Geometry check sheet. Reference: drawing and pictorial views, mm from the part's lowest x, y, z. Give positions to 0.01 mm unless a question says otherwise; leave off trailing zeros. Write each loop counter-clockwise with the first axis right and the second up, starting at its lowest first coordinate (ties: lowest second). Pieces come first, ordered by that corner, then holes. Notation, with made-up numbers: M 24.5,-33.75 L 65.5,-33.75 A19 ccw 65.5,2.25 Z; hole C 37.25,64.5 d10. An arc over 180 degrees is marked long. Answer as a JSON object with one key per item and string values.
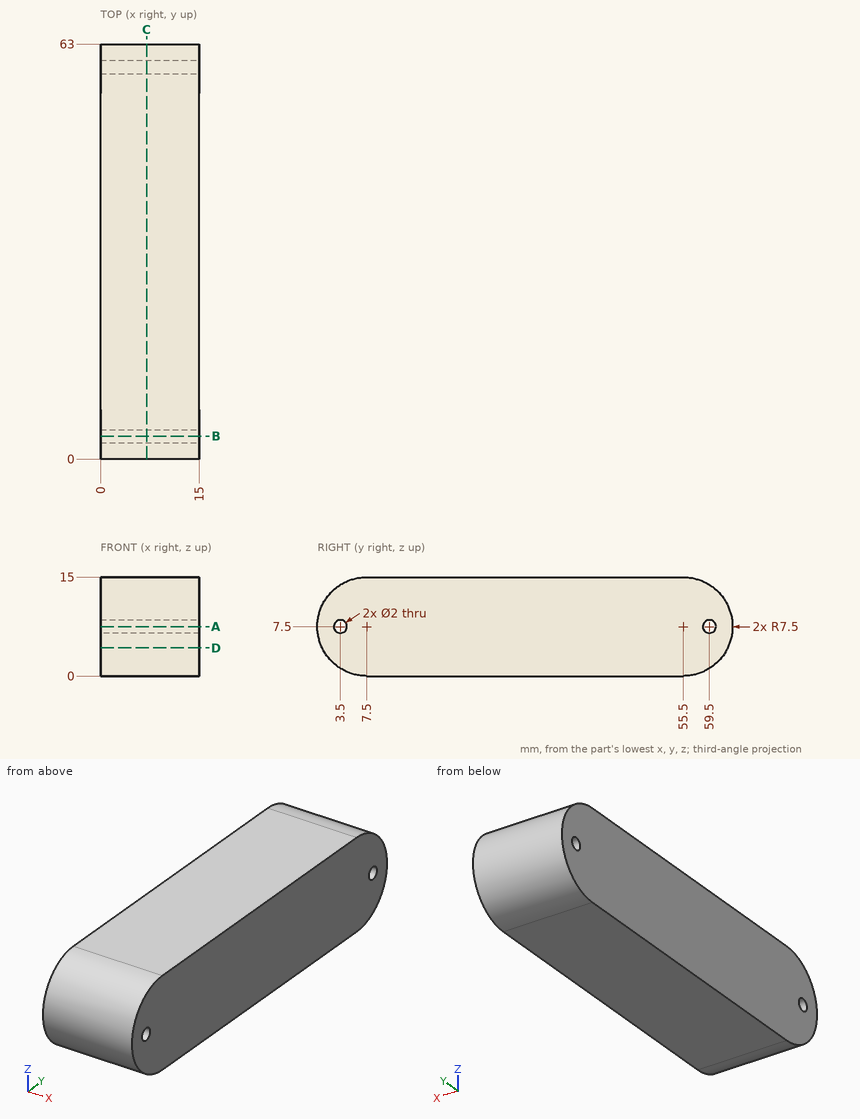
1) Section check C-C on x = 7. Record the boundary of the cut face in (y, z), and give its area (3 significant figures).
Completed:
{"outline": "M 7.5,0 L 55.5,0 A7.5 ccw 55.5,15 L 7.5,15 A7.5 ccw Z; hole C 3.5,7.5 d2; hole C 59.5,7.5 d2", "area": "890 mm2"}
2) Section check A-A on z = 7.5. Record the boundary of the cut face in (x, y).
Completed:
{"outline": "M 0,0 L 15,0 L 15,2.5 L 0,2.5 Z; M 0,4.5 L 15,4.5 L 15,58.5 L 0,58.5 Z; M 0,60.5 L 15,60.5 L 15,63 L 0,63 Z"}
3) Go/stop test with a flat-tipped pin: pin 1 (3 mm diameter, centred on x = 4.5, y = 32, fed in from -Z). Record where the tip stops, or that it passes through.
Completed:
{"pin 1": "stops at z = 0"}
4) Section check B-B on y = 3.5. Record the boundary of the cut face in (x, z), and give its area (3 significant figures).
Completed:
{"outline": "M 0,1.16 L 15,1.16 L 15,6.5 L 0,6.5 Z; M 0,8.5 L 15,8.5 L 15,13.84 L 0,13.84 Z", "area": "160 mm2"}
5) Section check D-D on z = 4.25. Record the boundary of the cut face in (x, y), and give its area (3 significant figures).
Completed:
{"outline": "M 0,0.74 L 15,0.74 L 15,62.26 L 0,62.26 Z", "area": "923 mm2"}
6) Thickness scan on L1, parallel to Y at x = 5, z = 7.5; L2, parallel to Y at x = 3.25, z = 8.25; L3, parallel to Z at x = 12.75, y = 4. Record the ranges inside material, lowest first.
Completed:
{"L1": "y = 0 to 2.5, 4.5 to 58.5, 60.5 to 63", "L2": "y = 0.04 to 2.84, 4.16 to 58.84, 60.16 to 62.96", "L3": "z = 0.87 to 6.63, 8.37 to 14.13"}
